from build123d import *

# Parameters (mm, degrees)
PAD003_DEPTH    = 3
SKETCH020_W     = 100
SKETCH020_H     = 80
POCKET004_DEPTH = 0.8
SKETCH021_R     = 3.7
PAD004_DEPTH    = 2.8
SKETCH022_R     = 3.7
PAD005_DEPTH    = 2
SKETCH023_R     = 1.7
POCKET005_DEPTH = 4
SKETCH024_R     = 1.7
POCKET006_DEPTH = 3
SKETCH025_W     = 6.5
SKETCH025_H     = 16.5
POCKET007_DEPTH = 3
FILLET_R        = 2
SKETCH026_R     = 1.7
POCKET008_DEPTH = 3
CHAMFER_SIZE    = 0.5
SKETCH036_W     = 60
SKETCH036_H     = 40
PAD006_DEPTH    = 2
SKETCH034_W     = 40
SKETCH034_H     = 1
POCKET009_DEPTH = 10
SKETCH035_W     = 40
SKETCH035_H     = 1
POCKET011_DEPTH = 10
SKETCH037_W     = 40
SKETCH037_H     = 1
POCKET010_DEPTH = 5


with BuildPart() as part:
    # Sketch033 → Pad003 (new body)
    with BuildSketch(Plane.XY):
        Polygon((-65.9, 40), (-57.9, 46), (57.9, 46), (65.9, 40), (65.9, -40), (57.9, -46), (-57.9, -46), (-65.9, -40), align=None)
    extrude(amount=PAD003_DEPTH)

    # Sketch020 → Pocket004 (cut)
    with BuildSketch(Plane.XY.offset(3)):
        with Locations((-8.9, 0)):
            Rectangle(SKETCH020_W, SKETCH020_H)
    extrude(amount=-POCKET004_DEPTH, mode=Mode.SUBTRACT)

    # Sketch021 (on Face15 of Pocket004) → Pad004 (join)
    with BuildSketch(Plane.XY.offset(2.2)):
        with Locations((-54.9, 36)):
            Circle(SKETCH021_R)
        with Locations((31.1, 36)):
            Circle(SKETCH021_R)
        with Locations((31.1, -22)):
            Circle(SKETCH021_R)
        with Locations((-54.9, -22)):
            Circle(SKETCH021_R)
    extrude(amount=PAD004_DEPTH)

    # Sketch022 (on Face5 of Pad004) → Pad005 (join)
    with BuildSketch(Plane.XY.offset(3)):
        with Locations((45.22, 37.46)):
            Circle(SKETCH022_R)
        with Locations((56.65, 37.46)):
            Circle(SKETCH022_R)
        with Locations((45.2, -37.46)):
            Circle(SKETCH022_R)
        with Locations((57.9, -37.46)):
            Circle(SKETCH022_R)
    extrude(amount=PAD005_DEPTH)

    # Sketch023 (on Face29 of Pad005) → Pocket005 (cut)
    with BuildSketch(Plane.XY.offset(5)):
        with Locations((-54.9, 36)):
            Circle(SKETCH023_R)
        with Locations((-54.9, -22)):
            Circle(SKETCH023_R)
        with Locations((31.1, -22)):
            Circle(SKETCH023_R)
        with Locations((31.1, 36)):
            Circle(SKETCH023_R)
        with Locations((45.22, 37.46)):
            Circle(SKETCH023_R)
        with Locations((56.65, 37.46)):
            Circle(SKETCH023_R)
        with Locations((45.2, -37.46)):
            Circle(SKETCH023_R)
        with Locations((57.9, -37.46)):
            Circle(SKETCH023_R)
    extrude(amount=-POCKET005_DEPTH, mode=Mode.SUBTRACT)

    # Sketch024 (on Face4 of Pocket005) → Pocket006 (cut)
    with BuildSketch(Plane(origin=(0, 0, 0), x_dir=(1, 0, 0), z_dir=(0, 0, -1))):
        with Locations((0, 43)):
            Circle(SKETCH024_R)
        with Locations((-62.65, 0)):
            Circle(SKETCH024_R)
        with Locations((62.65, 0)):
            Circle(SKETCH024_R)
        with Locations((0, -43)):
            Circle(SKETCH024_R)
    extrude(amount=-POCKET006_DEPTH, mode=Mode.SUBTRACT)

    # Sketch025 (on Face5 of Pocket006) → Pocket007 (cut)
    with BuildSketch(Plane.XY.offset(3)):
        with Locations((46.65, 0)):
            Rectangle(SKETCH025_W, SKETCH025_H)
    extrude(amount=-POCKET007_DEPTH, mode=Mode.SUBTRACT)

    # Fillet
    fillet_edges = [part.edges().sort_by_distance(p)[0] for p in [
        (43.4, 8.25, 1.5),
        (49.9, 8.25, 1.5),
        (43.4, -8.25, 1.5),
        (49.9, -8.25, 1.5),
    ]]
    fillet(fillet_edges, radius=FILLET_R)

    # Sketch026 (on Face22 of Fillet) → Pocket008 (cut)
    with BuildSketch(Plane.XY.offset(3)):
        with Locations((46.65, 11)):
            Circle(SKETCH026_R)
        with Locations((46.65, -11)):
            Circle(SKETCH026_R)
    extrude(amount=-POCKET008_DEPTH, mode=Mode.SUBTRACT)

    # Chamfer
    chamfer_edges = [part.edges().sort_by_distance(p)[0] for p in [
        (44.95, 11, 3),
        (44.95, -11, 3),
        (43.52, 37.46, 5),
        (54.95, 37.46, 5),
        (29.4, 36, 5),
        (-56.6, 36, 5),
        (-56.6, -22, 5),
        (29.4, -22, 5),
        (43.5, -37.46, 5),
        (56.2, -37.46, 5),
        (60.95, 0, 0),
        (-1.7, 43, 0),
        (-64.35, 0, 0),
        (-1.7, -43, 0),
    ]]
    chamfer(chamfer_edges, length=CHAMFER_SIZE)

    # Sketch036 (on Face1 of Chamfer) → Pad006 (join)
    with BuildSketch(Plane(origin=(0, 0, 0), x_dir=(1, 0, 0), z_dir=(0, 0, -1))):
        Rectangle(SKETCH036_W, SKETCH036_H)
    extrude(amount=PAD006_DEPTH)

    # Sketch034 (on Face13 of Pad006) → Pocket009 (cut)
    with BuildSketch(Plane.YZ.offset(30)):
        with Locations((0, -0.5)):
            Rectangle(SKETCH034_W, SKETCH034_H)
    extrude(amount=-POCKET009_DEPTH, mode=Mode.SUBTRACT)

    # Sketch035 (on Face76 of Pocket009) → Pocket011 (cut)
    with BuildSketch(Plane(origin=(-30, 0, 0), x_dir=(0, -1, 0), z_dir=(-1, 0, 0))):
        with Locations((0, -0.5)):
            Rectangle(SKETCH035_W, SKETCH035_H)
    extrude(amount=-POCKET011_DEPTH, mode=Mode.SUBTRACT)

    # Sketch037 (on Face76 of Pocket011) → Pocket010 (cut)
    with BuildSketch(Plane.XZ.offset(20)):
        with Locations((0, -0.5)):
            Rectangle(SKETCH037_W, SKETCH037_H)
    extrude(amount=-POCKET010_DEPTH, mode=Mode.SUBTRACT)


with BuildPart() as part_1:
    # Body003 placement: moved
    add(part.part.moved(Location((0, 0, 5))))


solid = part_1.part
Geometry: final body of the model. Coordinates: model frame, mm. A direction names the side the tool comes from. Coordinates: 2 decimals unless noted, no trailing zeros. Loops run counter-clockwise (first coordinate to the right, second up) from the corner with the lowest first, then second, coordinate; pieces in that order, holes last. Notation, with made-up numbers: M 80.5,7.25 L 115.5,7.25 A21 cw 115.5,43.25 Z; hole C 72,-5.75 d5. An arc over 180 degrees is marked long. One line per item, written item: value. Start each with the question number.
1) Material intervals for L1, parallel to Y at x = -54.9, z = 7.7; L2, parallel to Y at x = 0, z = 6.1; L3, parallel to X at y = 0, z = 6.5, sorted ascending. Write a range as from..to.
2) Reachability of faces 1 (the flat face through (7, -18, 4)), 2 (the flat face through (58, -37, 6)), 3 (the flat face through (47, -39, 10)) from +Z, -Z, +X, -X, +Y, -Y: full face, straight path, thin tool, end or side. Return the list, or none.
3) Cut plane D-D (y = 24). Return loops of the section in (x, z).
4) Pin query (flat end, axial travel): P1, Ø2, axis at x = -47.5, y = -15, coming from the -Z side; P2, Ø1.1, axis at x = 6.5, z = 3.5, coming from the -Y side; P3, Ø1, axis at x = 6.5, y = 13, coming from the +Z side; P4, Ø2, axis at x = -14.5, y = 20.5, coming from the -Z side. Return the tip coordinate at first contact, or that it passes through.
5) Draft query along Y for faces 4 (the cylindrical face through (29.4, -21.93, 7.77)), 5 (the flat face through (-53, -24, 10)), 6 (the cylindrical face through (-0.37, -41.34, 6.73)), 7 (the flat face through (-61.956, 42.958, 6.479)). Return one class per face: released by +Y, released by -Y, zero draft, split by the parting line, or undercut.
6) Cut plane A-A (x = -25). Return loops of the section in (y, z), then the cut area to 3 significant figures.
7) Cut plane C-C (y = 11). Return loops of the section in (x, z).
8) Cut plane B-B (y = -4.5). Return loops of the section in (x, z).
Evaluation:
1. L1: -46..-40, -25.7..-23.7, -20.3..-18.3, 32.3..34.3, 37.7..39.7, 40..46
1. L2: -46..-44.7, -41.3..41.3, 44.7..46
1. L3: -65.9..-64.35, -60.95..43.4, 49.9..60.95, 64.35..65.9
2. face 1: -Y
2. face 2: +Z
2. face 3: +Z, +X, -X, +Y, -Y
3. outline: M -65.9,5 L 65.9,5 L 65.9,8 L 41.1,8 L 41.1,7.2 L -58.9,7.2 L -58.9,8 L -65.9,8 Z
4. P1: z = 5
4. P2: y = -20
4. P3: z = 7.2
4. P4: z = 3
5. face 4: undercut
5. face 5: zero draft
5. face 6: undercut
5. face 7: released by +Y
6. outline: M -46,5 L 46,5 L 46,8 L 40,8 L 40,7.2 L -40,7.2 L -40,8 L -46,8 Z; M -20,3 L 20,3 L 20,4 L -20,4 Z
6. area: 252 mm^2
7. outline: M -65.9,5 L -20,5 L -20,4 L -30,4 L -30,3 L 30,3 L 30,4 L 20,4 L 20,5 L 44.95,5 L 44.95,7.5 L 44.45,8 L 41.1,8 L 41.1,7.2 L -58.9,7.2 L -58.9,8 L -65.9,8 Z; M 48.35,5 L 65.9,5 L 65.9,8 L 48.85,8 L 48.35,7.5 Z
8. outline: M -65.9,5 L -20,5 L -20,4 L -30,4 L -30,3 L 30,3 L 30,4 L 20,4 L 20,5 L 43.4,5 L 43.4,8 L 41.1,8 L 41.1,7.2 L -58.9,7.2 L -58.9,8 L -65.9,8 Z; M 49.9,5 L 65.9,5 L 65.9,8 L 49.9,8 Z
